Here's how the part is built. I have some questions about the finished solid (model axes, mm). A direction names the side the tool comes from. Round coordinates to 2 decimals unless told otherwise and drop trailing zeros. Order: outer loops, then holes, each group sorted by start corner. A loop starts at its lowest first (then second) coordinate and runs counter-clockwise, first axis right, second up. Notation, with made-up numbers: M 21,85 L 40,85 A25 cw 40,105 Z; hole C 22.5,69 d5. An arc over 180 degrees is marked long. Write item = value, one per line. Start each with the question number.
Item 1: For faces 1 (the face through (-4, 0, 95)), 2 (the face through (1, 0, 35)), which set-ups out of +Z, -Z, +X, -X, +Y, -Y let a thin tool reach every point of the face, with its end or its side?
Item 2: We'd pull the mould along X, two halves only. Please class faces 3 (the face through (-49.75, -0.08, 47.23)), 4 (the face through (-4, 6, 1)), 5 (the face through (-305, 0, -1)): pulls with the +X half, pulls with the -X half, needs draft (parallel to the pull), parting line crosses it, or undercut.
Item 3: Please list where these lines run through material, in increasing order: L1, parallel to Z at x = 289, y = -2.5; L2, parallel to X at y = 0.25, z = -65; L3, parallel to X at y = 4, z = 48.
Item 4: I want a section at A-A, the plane y = -2.25. List the corners of the cut face in (x, z) for me.
```python
from build123d import *

# Parameters (mm, degrees)
F0_W     = 610
F0_H     = 190
F0_R     = 1.5
F1_DEPTH = 6


with BuildPart() as f1:
    # F0 (on Front) → F1 (new body, symmetric)
    with BuildSketch(Plane.XZ):
        Rectangle(F0_W, F0_H)
        with Locations((-289, -65)):
            Circle(F0_R, mode=Mode.SUBTRACT)
        with Locations((289, -65)):
            Circle(F0_R, mode=Mode.SUBTRACT)
        with Locations((-289, 50)):
            Circle(F0_R, mode=Mode.SUBTRACT)
        with BuildLine():
            ThreePointArc((37.7469517291, 60), (50.2469517291, 47.5), (37.7469517291, 35))
            Line((37.7469517291, 35), (-37.2530482709, 35))
            ThreePointArc((-37.2530482709, 35), (-49.7530482709, 47.5), (-37.2530482709, 60))
            Line((-37.2530482709, 60), (37.7469517291, 60))
        make_face(mode=Mode.SUBTRACT)
        with Locations((289, 50)):
            Circle(F0_R, mode=Mode.SUBTRACT)
    extrude(amount=F1_DEPTH, both=True)


solid = f1.part
```
Filled in:
q1.face_1 = +Z, +X, -X, +Y, -Y
q1.face_2 = +Y, -Y
q2.face_3 = undercut
q2.face_4 = needs draft
q2.face_5 = pulls with the -X half
q3.L1 = -95 to -66.5, -63.5 to 48.5, 51.5 to 95
q3.L2 = -305 to -290.5, -287.5 to 287.5, 290.5 to 305
q3.L3 = -305 to -49.74, 50.24 to 305
q4.outline = M -305,-95 L 305,-95 L 305,95 L -305,95 Z; hole C -289,-65 d3; hole C -289,50 d3; hole M -37.25,35 L 37.75,35 A12.5 ccw 37.75,60 L -37.25,60 A12.5 ccw Z; hole C 289,-65 d3; hole C 289,50 d3
